```python
from build123d import *

# Parameters (mm, degrees)
F1_W     = 115.4
F1_H     = 115.4
F1_W_2   = 64.6
F1_H_2   = 64.6
F2_DEPTH = 25.4
F0_W     = 25.4
F0_H     = 25.4
F3_DEPTH = 250
F4_W     = 25.4
F4_H     = 25.4
F4_W_2   = 64.6
F4_H_2   = 64.6
F5_DEPTH = 25


with BuildPart() as f2:
    # F1 (on Front) → F2 (new body)
    with BuildSketch(Plane.XZ):
        Rectangle(F1_W, F1_H)
        Rectangle(F1_W_2, F1_H_2, mode=Mode.SUBTRACT)
    extrude(amount=-F2_DEPTH)

    # F0 (on Front) → F3 (join)
    with BuildSketch(Plane.XZ):
        with Locations((45, 45)):
            Rectangle(F0_W, F0_H)
        with Locations((-45, 45)):
            Rectangle(F0_W, F0_H)
        with Locations((-45, -45)):
            Rectangle(F0_W, F0_H)
        with Locations((45, -45)):
            Rectangle(F0_W, F0_H)
    extrude(amount=F3_DEPTH)

    # F4 (on face) → F5 (join)
    with BuildSketch(Plane.XZ.offset(250)):
        with Locations((-45, 45)):
            Rectangle(F4_W, F4_H)
        Polygon((57.7, 57.7), (-32.3, 57.7), (-32.3, 32.3), (-57.7, 32.3), (-57.7, -57.7), (57.7, -57.7), align=None)
        Rectangle(F4_W_2, F4_H_2, mode=Mode.SUBTRACT)
    extrude(amount=F5_DEPTH)


solid = f2.part
```
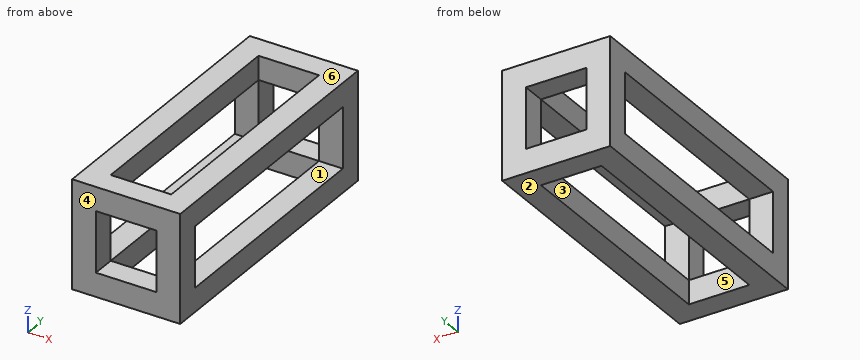
For this review, take the finished solid that the model builds, in its own axes (mm). Face numbers are marked on the shaded views. A direction names the side the tool comes from. Coordinates: 2 decimals unless noted, no trailing zeros. Order: outer loops, then holes, each group sorted by start corner. A loop starts at its lowest first (then second) coordinate and runs counter-clockwise, first axis right, second up. Notation, with made-up numbers: (72.5, -29) -> (119.5, -29) arc R11 ccw to (119.5, -10) -> close; hole circle Ø10 at (13, 24). An arc over 180 degrees is marked (long way). Use CSV: the item, a comma, the result in double quotes. Start each with the question number.
Item 1: Wall thickness on probe 1 along Y at (x, z) = (-11.5, 42); probe 2 along Z at (x, y) = (-51.5, -246.5): over which ranges is each line inside the solid? List them lowest first.
Item 2: We need section A-A, the plane x = -5. Give the boundary of the cut face in (y, z), then the cut area to 3 significant figures.
Item 3: Draft analysis for pull direction Y (two halves, no side actions). For the marked faces 4, 5 and 6, state which applies: pulls with the +Y half, pulls with the -Y half, needs draft (parallel to the pull), parting line crosses it, or undercut.
Item 4: We need section C-C, the plane z = 43.5. Give the boundary of the cut face in (x, y), then the cut area to 3 significant figures.
Item 5: For the marked faces 1, 2 and 3, list the 3-axis set-ups (+Z, -Z, +X, -X, +Y, -Y) from which the entire face can be reached by the end or side of a thin tool; tool diameter is ignored.
Item 6: We need section D-D, the plane y = -253. Give the boundary of the cut face in (x, z).
Item 7: We need section B-B, the plane y = -67. Give the boundary of the cut face in (x, z), then the cut area to 3 significant figures.
Derived:
1,probe 1,"y = -275 to -250, 0 to 25.4"
1,probe 2,"z = -57.7 to -32.3, 32.3 to 57.7"
2,outline,"(-275, -57.7) -> (-250, -57.7) -> (-250, -32.3) -> (-275, -32.3) -> close; (-275, 32.3) -> (-250, 32.3) -> (-250, 57.7) -> (-275, 57.7) -> close; (0, -57.7) -> (25.4, -57.7) -> (25.4, -32.3) -> (0, -32.3) -> close; (0, 32.3) -> (25.4, 32.3) -> (25.4, 57.7) -> (0, 57.7) -> close"
2,area,"2,560 mm^2"
3,face 4,"pulls with the -Y half"
3,face 5,"undercut"
3,face 6,"needs draft"
4,outline,"(-57.7, -275) -> (57.7, -275) -> (57.7, 25.4) -> (-57.7, 25.4) -> close; hole (-32.3, -250) -> (32.3, -250) -> (32.3, 0) -> (-32.3, 0) -> close"
4,area,"18,500 mm^2"
5,face 1,"+X, -X"
5,face 2,"-Z, +X, -X, +Y, -Y"
5,face 3,"+Z, -Z"
6,outline,"(-57.7, -57.7) -> (57.7, -57.7) -> (57.7, 57.7) -> (-57.7, 57.7) -> close; hole (-32.3, -32.3) -> (32.3, -32.3) -> (32.3, 32.3) -> (-32.3, 32.3) -> close"
7,outline,"(-57.7, -57.7) -> (-32.3, -57.7) -> (-32.3, -32.3) -> (-57.7, -32.3) -> close; (-57.7, 32.3) -> (-32.3, 32.3) -> (-32.3, 57.7) -> (-57.7, 57.7) -> close; (32.3, -57.7) -> (57.7, -57.7) -> (57.7, -32.3) -> (32.3, -32.3) -> close; (32.3, 32.3) -> (57.7, 32.3) -> (57.7, 57.7) -> (32.3, 57.7) -> close"
7,area,"2,580 mm^2"
